CAD build for the part. Positions are in the model's coordinates, mm. A direction names the side the tool comes from. Give positions to 0.01 mm unless a question says otherwise; leave off trailing zeros. Order: outer loops, then holes, each group sorted by start corner. A loop starts at its lowest first (then second) coordinate and runs counter-clockwise, first axis right, second up. Notation, with made-up numbers: (-22.5, 48.25) -> (-17.5, 48.25) arc R19 cw to (-17.5, 72.25) -> close; hole circle Ø6 at (-7.75, 45.5). An arc over 180 degrees is marked (long way). Use one line per item in the form item = value. Start each with the question number.
1) Cut at D-D, the plane y = 26.5. Give the cut face in (x, z).
2) Tool access for faces 1 (the face through (7, 24, -13)), 2 (the face through (-42, 17, -9)), 3 (the face through (5.6, 14, 0)), 4 (the face through (7, 6, -11)): list every direction of +Z, -Z, +X, -X, +Y, -Y with a clear straight run to the whole face (end or side of a thin tool).
3) Drop flat-ended pins along their axis: P1, Ø1.5, axis at y = 16, z = -8.5, coming from the +X side; P2, Ø1, axis at x = 11.5, z = 15.5, coming from the +Y side; P3, Ø1.2, axis at x = -48.5, z = -15.5, coming from the +Y side. Give the stop position or say it passes through.
4) Mould opens along Z. For faces 5 (the face through (1, 0, 0)), 6 (the face through (28.35, 18.29, 1.27)), 7 (the face through (1, 20, 25)) say: pulls with the +Z half, pulls with the -Z half, needs draft (parallel to the pull), parting line crosses it, or undercut.
5) Cut at A-A, the plane y = 12.5. Give the cut face in (x, z).
6) Cut at B-B, the plane x = -39.5. Give the cut face in (y, z), and give its area (3 significant figures).
7) Cut at C-C, the plane z = 17.5. Give the cut face in (x, y).
8) Probe line 1 (X direction, y = 23.5, z = -13.5); line 2 (Z direction, x = 30, y = 10.5); line 3 (Y direction, x = 28, z = 0). List the from-to ranges inside material, lowest first.
Autodesk Inventor part; units mm, degrees
ref_plane "YZ Plane" through (0, 0, 0) normal (1, 0, 0) x (0, 1, 0)
ref_plane "XZ Plane" through (0, 0, 0) normal (0, 1, 0) x (-1, 0, 0)
ref_plane "XY Plane" through (0, 0, 0) normal (0, 0, 1) x (1, 0, 0)
sketch "Sketch1" plane through (0, 0, 0) normal (0, 1, 0) x (-1, 0, 0)
  line L0 (50, -25) -> (-50, -25)
  line L1 (-50, -25) -> (-50, 25)
  line L2 (-50, 25) -> (50, 25)
  line L3 (50, 25) -> (50, -25)
  point P0 (0, 0)
  dimension "d0" = 100
  dimension "d1" = 50
  dimension "d2" = 25
  dimension "d3" = 50
extrude "Extrusion1" add sketch "Sketch1" along normal blind 4
sketch "Sketch2" plane through (0, 4, 0) normal (0, 1, 0) x (1, 0, 0)
  line L0 (50, -25) -> (-50, -25)
  line L1 (-50, -25) -> (-50, -21)
  line L2 (-50, -21) -> (50, -21)
  line L3 (50, -21) -> (50, -25)
  line L4 (50, 25) -> (-50, 25)
  line L5 (-50, 25) -> (-50, 21)
  line L6 (-50, 21) -> (50, 21)
  line L7 (50, 21) -> (50, 25)
  point P0 (0, 0)
  dimension "d7" = 100
  dimension "d8" = 4
  dimension "d10" = 4
extrude "Extrusion2" add sketch "Sketch2" along normal blind 36
sketch "Sketch3" plane through (0, 4, 0) normal (0, 1, 0) x (1, 0, 0)
  line L0 (50, 21) -> (-50, 21)
  line L1 (28.6, 21) -> (25.6, 21)
  line L2 (25.6, 21) -> (25.6, -21)
  line L3 (25.6, -21) -> (28.6, -21)
  line L4 (28.6, -21) -> (28.6, 21)
  line L5 (50, -21) -> (50, 21)
  line L6 (50, -21) -> (-50, -21)
  point P0 (0, 0)
  dimension "d15" = 21.4
  dimension "d16" = 0
  dimension "d17" = 3
extrude "Extrusion3" add sketch "Sketch3" along normal blind 32 contours L4 L3 L2 L0
sketch "Sketch4" plane through (28.6, 4, 21) normal (1, 0, 0) x (0, 0, -1)
  circle A0 centre (21, 20) radius 5
  line L0 (0, 0) -> (42, 0)
  line L1 (0, 0) -> (0, 36)
  circle A1 centre (13.6, 20) radius 1.25
  point P0 (21, -4)
  dimension "d20" = 10
  dimension "d22" = 21
  dimension "d23" = 2.5
  dimension "d24" = 7.4
  dimension "d28" = 20
  dimension "d29" = 20
extrude "Extrusion4" cut sketch "Sketch4" against normal up to next
sketch "Sketch5" plane through (28.6, 4, 21) normal (1, 0, 0) x (0, 0, -1)
  circle A0 centre (21, 20) radius 5
  circle A1 centre (21, 20) radius 5.85
  point P0 (21, -4)
  dimension "d30" = 11.7
extrude "Extrusion5" cut sketch "Sketch5" against normal blind 0.5
sketch "Sketch6" plane through (0, 4, 0) normal (0, 1, 0) x (1, 0, 0)
  line L0 (8.6, -21) -> (5.6, -21)
  line L1 (5.6, -21) -> (5.6, 21.1393)
  line L2 (5.6, 21.1393) -> (8.6, 21.1393)
  line L3 (8.6, 21.1393) -> (8.6, -21)
  line L4 (25.6, -21) -> (25.6, 21)
  line L5 (50, -21) -> (-50, -21)
  line L6 (-50, 21) -> (-50, -21)
  point P0 (0, 0)
  dimension "d34" = 3
  dimension "d35" = 0
  dimension "d52" = 55.6
extrude "Extrusion6" add sketch "Sketch6" along normal blind 20
sketch "Sketch7" plane through (5.6, 4, -21) normal (-1, 0, 0) x (0, 0, 1)
  circle A0 centre (21, 20) radius 5
  circle A1 centre (21, 20) radius 5
  point P0 (21, -4)
  dimension "d38" = 10
extrude "Extrusion7" cut sketch "Sketch7" against normal up to next
sketch "Sketch8" plane through (5.6, 4, -21) normal (-1, 0, 0) x (0, 0, 1)
  line L0 (8, 13) -> (17, 13)
  line L1 (17, 13) -> (17, 10)
  line L2 (17, 10) -> (8, 10)
  line L3 (8, 10) -> (8, 13)
  line L4 (0, 0) -> (0, 36)
  line L5 (0, 0) -> (42, 0)
  point P0 (21, -4)
  dimension "d41" = 8
  dimension "d42" = 9
  dimension "d43" = 10
  dimension "d44" = 3
extrude "Extrusion8" add sketch "Sketch8" along normal blind 6.1
sketch "Sketch10" plane through (0, 4, 0) normal (0, 1, 0) x (1, 0, 0)
  line L0 (-50, -21) -> (-50, -25)
  line L1 (-50, 21) -> (50, 21)
  line L2 (-50, -21) -> (-46, -21)
  line L3 (-46, -21) -> (-46, 21)
  line L4 (-46, 21) -> (-50, 21)
  line L5 (-50, 21) -> (-50, -21)
  point P0 (0, 0)
  dimension "d53" = 4
extrude "Extrusion10" add sketch "Sketch10" along normal blind 20
sketch "Sketch11" plane through (-50, 0, -25) normal (-1, 0, 0) x (0, 0, 1)
  circle A0 centre (25, 24) radius 7.5
  point P0 (25, 0)
  dimension "d56" = 15
extrude "Extrusion11" cut sketch "Sketch11" against normal up to surface (4 mm away)
sketch "Sketch12" plane through (-46, 4, 21) normal (1, 0, 0) x (0, 0, -1)
  line L0 (34, 13) -> (25, 13)
  line L1 (25, 13) -> (25, 10)
  line L2 (25, 10) -> (34, 10)
  line L3 (34, 10) -> (34, 13)
  line L4 (42, 20) -> (42, 36)
  line L5 (-4, -4) -> (46, -4)
  point P0 (21, -4)
  dimension "d59" = 9
  dimension "d60" = 8
  dimension "d61" = 3
  dimension "d62" = 14
extrude "Extrusion12" add sketch "Sketch12" along normal blind 8.5
sketch "Sketch9" plane through (5.6, 17, -4) normal (0, 1, 0) x (1, 0, 0)
  line L0 (0, 17) -> (0, 1)
  line L1 (-51.6, 3.5) -> (-51.6, 17)
  line L2 (-51.6, 9) -> (-43.1, 9)
  line L3 (-45.1, 5.5) -> (-45.1, 3.5) construction
  line L4 (-46.1, 5.5) -> (-46.1, 3.5)
  line L5 (-44.1, 3.5) -> (-44.1, 5.5)
  arc A0 (-44.1, 5.5) -> (-46.1, 5.5) centre (-45.1, 5.5) ccw
  arc A1 (-46.1, 3.5) -> (-44.1, 3.5) centre (-45.1, 3.5) ccw
  line L6 (-4.1, 5.5) -> (-4.1, 3.5) construction
  line L7 (-5.1, 5.5) -> (-5.1, 3.5)
  line L8 (-3.1, 3.5) -> (-3.1, 5.5)
  arc A2 (-3.1, 5.5) -> (-5.1, 5.5) centre (-4.1, 5.5) ccw
  arc A3 (-5.1, 3.5) -> (-3.1, 3.5) centre (-4.1, 3.5) ccw
  line L9 (0, 9) -> (-6.1, 9)
  point P0 (-5.6, -4)
  point P1 (-45.1, 4.5)
  point P2 (-4.1, 4.5)
  dimension "d68" = 2
  dimension "d70" = 2
  dimension "d71" = 6.5
  dimension "d72" = 2
  dimension "d73" = 2
  dimension "d74" = 4.1
  dimension "d75" = 4.5
  dimension "d76" = 4.5
extrude "Extrusion9" cut sketch "Sketch9" against normal blind 3
sketch "Sketch13" plane through (0, 40, 0) normal (0, 1, 0) x (1, 0, 0)
  line L0 (-48, 21) -> (-46, 21)
  line L1 (-46, 21) -> (-46, 23)
  line L2 (-46, 23) -> (-48, 23)
  line L3 (-48, 23) -> (-48, 21)
  line L4 (-50, 21) -> (50, 21)
  line L5 (-50, 25) -> (-50, 21)
  line L6 (-48, -23) -> (-46, -23)
  line L7 (-46, -23) -> (-46, -21)
  line L8 (-46, -21) -> (-48, -21)
  line L9 (-48, -21) -> (-48, -23)
  line L10 (-50, -21) -> (-50, -25)
  line L11 (50, -21) -> (-50, -21)
  point P0 (0, 0)
  dimension "d77" = 2
  dimension "d78" = 2
  dimension "d79" = 0
  dimension "d80" = 2
  dimension "d81" = 2
  dimension "d82" = 2
  dimension "d83" = 2
  dimension "d84" = 0
extrude "Extrusion13" cut sketch "Sketch13" against normal up to surface (16 mm away)
sketch "Sketch14" plane through (28.6, 4, 21) normal (1, 0, 0) x (0, 0, -1)
  line L0 (0, 0) -> (42, 0)
  line L1 (42, 0) -> (32, 0)
  line L2 (32, 0) -> (32, 5)
  line L3 (32, 5) -> (42, 5)
  line L4 (42, 5) -> (42, 0)
  point P0 (21, -4)
  dimension "d87" = 10
  dimension "d88" = 5
extrude "Extrusion14" cut sketch "Sketch14" against normal up to surface (23 mm away)
properties part number "BoxBase"
Result:
q1.outline = (-50, -25) -> (50, -25) -> (50, -21) -> (28.6, -21) -> (28.6, -5.29) -> (28.1, -5.29) -> (28.1, -4.33) -> (25.6, -4.33) -> (25.6, -21) -> (-46, -21) -> (-46, -23) -> (-48, -23) -> (-48, -21) -> (-50, -21) -> close; (-50, 21) -> (-48, 21) -> (-48, 23) -> (-46, 23) -> (-46, 21) -> (25.6, 21) -> (25.6, 4.33) -> (28.1, 4.33) -> (28.1, 5.29) -> (28.6, 5.29) -> (28.6, 21) -> (50, 21) -> (50, 25) -> (-50, 25) -> close
q2.face_1 = -X, +Y
q2.face_2 = +Y
q2.face_3 = none
q2.face_4 = +X
q3.P1 = 28.6
q3.P2 = 4
q3.P3 = 24
q4.face_5 = needs draft
q4.face_6 = undercut
q4.face_7 = pulls with the +Z half
q5.outline = (-50, -25) -> (50, -25) -> (50, -21) -> (28.6, -21) -> (28.6, 21) -> (50, 21) -> (50, 25) -> (-50, 25) -> close; hole (-46, -21) -> (5.6, -21) -> (5.6, 21) -> (-46, 21) -> close; hole (8.6, -21) -> (25.6, -21) -> (25.6, 21) -> (8.6, 21) -> close
q6.outline = (0, -25) -> (40, -25) -> (40, -21) -> (4, -21) -> (4, 21) -> (40, 21) -> (40, 25) -> (0, 25) -> close; (14, -13) -> (17, -13) -> (17, -10.5) -> (14, -10.5) -> close; (14, -6.5) -> (17, -6.5) -> (17, -4) -> (14, -4) -> close
q6.area = 503 mm²
q7.outline = (-50, 0) -> (50, 0) -> (50, 4) -> (28.6, 4) -> (28.6, 36) -> (25.6, 36) -> (25.6, 4) -> (8.6, 4) -> (8.6, 24) -> (5.6, 24) -> (5.6, 4) -> (-46, 4) -> (-46, 24) -> (-50, 24) -> close
q8.line_1 = -50 to -46, 5.6 to 8.6, 25.6 to 28.6
q8.line_2 = -25 to -21, 21 to 25
q8.line_3 = 0 to 19, 29 to 36
